from build123d import *

# Parameters (mm, degrees)
ESQUISSE1_W             = 37
ESQUISSE1_H             = 20
ESQUISSE1_R             = 2.05
ESQUISSE1_R_2           = 1.6
BOSS_EXTRU_1_DEPTH      = 2.5
ESQUISSE3_R             = 1.6
ENL_V_MAT_EXTRU_1_DEPTH = 1
ESQUISSE5_W             = 2.5
ESQUISSE5_H             = 20
ENL_V_MAT_EXTRU_3_DEPTH = 39.408983324


with BuildPart() as part:
    # Esquisse1 → Boss.-Extru.1 (new body)
    with BuildSketch(Plane.XY):
        Rectangle(ESQUISSE1_W, ESQUISSE1_H)
        with Locations((-12, 6)):
            Circle(ESQUISSE1_R, mode=Mode.SUBTRACT)
        with Locations((-12, -6)):
            Circle(ESQUISSE1_R, mode=Mode.SUBTRACT)
        with Locations((15.5, 0)):
            Circle(ESQUISSE1_R, mode=Mode.SUBTRACT)
        with Locations((3.4, -1.5)):
            Circle(ESQUISSE1_R_2, mode=Mode.SUBTRACT)
        with BuildLine():
            Line((-2.311989303, -5.883283951), (1.258004011, -3.143731482))
            ThreePointArc((1.258004011, -3.143731482), (4.267841424, 1.056726669), (4.098811422, -4.107999731))
            Line((4.098811422, -4.107999731), (5.263497125, -8.454665949))
            ThreePointArc((5.263497125, -8.454665949), (5.714243798, 5.317937785), (-2.311989303, -5.883283951))
        make_face(mode=Mode.SUBTRACT)
    boss_extru_1 = extrude(amount=BOSS_EXTRU_1_DEPTH)

    # Esquisse3 → Enlèv. mat.-Extru.1 (cut)
    # profile 1 of 2: a face of its own
    with BuildSketch(Plane(origin=(0, 0, 0), x_dir=(-1, 0, 0), z_dir=(0, 0, -1))):
        with BuildLine():
            Line((2.311989303, -5.883283951), (-1.258004011, -3.143731482))
            ThreePointArc((-1.258004011, -3.143731482), (-4.267841424, 1.056726669), (-4.098811422, -4.107999731))
            Line((-4.098811422, -4.107999731), (-5.263497125, -8.454665949))
            ThreePointArc((-5.263497125, -8.454665949), (-5.714243798, 5.317937785), (2.311989303, -5.883283951))
        make_face()
    # profile 2 of 2: a face of its own
    with BuildSketch(Plane(origin=(0, 0, 0), x_dir=(-1, 0, 0), z_dir=(0, 0, -1))):
        with BuildLine():
            Line((-4.681154273, -6.28133284), (0.526992646, -4.513507717))
            Line((0.526992646, -4.513507717), (-1.258004011, -3.143731482))
            ThreePointArc((-1.258004011, -3.143731482), (-4.267841424, 1.056726669), (-4.098811422, -4.107999731))
            Line((-4.098811422, -4.107999731), (-4.681154273, -6.28133284))
        make_face()
        with Locations((-3.4, -1.5)):
            Circle(ESQUISSE3_R, mode=Mode.SUBTRACT)
    enl_v_mat_extru_1 = extrude(amount=-ENL_V_MAT_EXTRU_1_DEPTH, mode=Mode.SUBTRACT)

    # Symétrie1: Boss.-Extru.1, Enlèv. mat.-Extru.1 across plane
    add(boss_extru_1.mirror(Plane(origin=(18.5, 0, 0), x_dir=(0, 0, 1), z_dir=(1, 0, 0))))
    add(enl_v_mat_extru_1.mirror(Plane(origin=(18.5, 0, 0), x_dir=(0, 0, 1), z_dir=(1, 0, 0))), mode=Mode.SUBTRACT)

    # Esquisse5 → Enlèv. mat.-Extru.3 (cut, through all)
    with BuildSketch(Plane(origin=(18.5, 0, 0), x_dir=(0, 0, -1), z_dir=(1, 0, 0))):
        with Locations((-1.25, 0)):
            Rectangle(ESQUISSE5_W, ESQUISSE5_H)
    extrude(amount=-ENL_V_MAT_EXTRU_3_DEPTH, mode=Mode.SUBTRACT)


solid = part.part
Check sheet for the modelled part. Datum: model origin and axes. Units: mm. A direction names the side the tool comes from. Round coordinates to 2 decimals unless told otherwise and drop trailing zeros. Order: outer loops, then holes, each group sorted by start corner. A loop starts at its lowest first (then second) coordinate and runs counter-clockwise, first axis right, second up.
Q1. Cross-section at D-D, the plane x = 49. Enter the section's corners in (y, z), plus the area to 3 significant figures.
Filled sheet:
outline: (-10, 0) - (-8.05, 0) - (-8.05, 2.5) - (-10, 2.5) - close; (-3.95, 0) - (3.95, 0) - (3.95, 2.5) - (-3.95, 2.5) - close; (8.05, 0) - (10, 0) - (10, 2.5) - (8.05, 2.5) - close
area: 29.5 mm2
Q2. Cross-section at C-C, the plane y = 0.5. Enter the section's corners in (x, z).
Filled sheet:
outline: (18.5, 0) - (19.51, 0) - (19.51, 2.5) - (18.5, 2.5) - close; (23.49, 0) - (26.68, 0) - (26.68, 2.5) - (23.49, 2.5) - close; (31.79, 1) - (35.41, 1) - (35.41, 2.5) - (31.79, 2.5) - close; (40.52, 0) - (55.5, 0) - (55.5, 2.5) - (40.52, 2.5) - close
Q3. Draft check along X on faces 1 (the face through (41, 0, 0)), 2 (the face through (33.4, -3.3, 1)), 3 (the face through (18.5, 0, 1)). Enter one of: pulls with the +X half, pulls with the -X half, needs draft (parallel to the pull), parting line crosses it, or undercut.
Filled sheet:
face 1: needs draft
face 2: undercut
face 3: pulls with the -X half
Q4. Depth check by flat-ended pin: P1, Ø3.5, axis at x = 49, y = 6, coming from the -Z side; P2, Ø3.5, axis at x = 35, y = -2, coming from the -Z side. Enter the tip coordinate at first touch or a pass-through.
Filled sheet:
P1: passes through
P2: stops at z = 1
Q5. Cross-section at A-A, the plane x = 21.5. Enter the section's corners in (y, z).
Filled sheet:
outline: (-10, 0) - (-2.05, 0) - (-2.05, 2.5) - (-10, 2.5) - close; (2.05, 0) - (10, 0) - (10, 2.5) - (2.05, 2.5) - close
Q6. Set-up check for faces 4 (the face through (34.89, -5.41, 0.49)), 5 (the face through (37.9, -4.8, 1.5)), 6 (the face through (37, 10, 1)): record each of +Z, -Z, +X, -X, +Y, -Y from which the full face is reachable in a straight line by a thin tool's end or side.
Filled sheet:
face 4: -Z
face 5: +Z, -Z
face 6: +Z, -Z, +X, -X, +Y
Q7. Scan lines: L1, parallel to Y at x = 33.6, z = 1.2; L2, parallel to Y at x = 21.5, z = 1.2; L3, parallel to Y at x = 49, z = 1.1. Record each from-to range of solid material in increasing order.
Filled sheet:
L1: y = -10 to -3.1, 0.1 to 1.2, 5.7 to 10
L2: y = -10 to -2.05, 2.05 to 10
L3: y = -10 to -8.05, -3.95 to 3.95, 8.05 to 10
Q8. Cross-section at B-B, the plane z = 1.5. Enter the section's corners in (x, y), plus the area to 3 significant figures.
Filled sheet:
outline: (18.5, -10) - (55.5, -10) - (55.5, 10) - (18.5, 10) - close; hole circle Ø4.1 at (21.5, 0); hole (31.74, -8.45) - (32.9, -4.11) arc R2.7 cw (long way) to (35.74, -3.14) - (39.31, -5.88) arc R7.2 ccw (long way) to start; hole circle Ø3.2 at (33.6, -1.5); hole circle Ø4.1 at (49, -6); hole circle Ø4.1 at (49, 6)
area: 579 mm2
